from build123d import *

# Parameters (mm, degrees)
SKETCH1_R           = 2.375
BOSS_EXTRUDE1_DEPTH = 22.5
SKETCH2_R           = 1.6
BOSS_EXTRUDE2_DEPTH = 0.6
SKETCH3_R           = 2.375
BOSS_EXTRUDE3_DEPTH = 4.4


with BuildPart() as part:
    # Sketch1 → Boss-Extrude1 (new body)
    with BuildSketch(Plane.XY):
        with Locations(Location((0, 0, 0), (0, 0, 180))):
            Circle(SKETCH1_R)
    boss_extrude1 = extrude(amount=BOSS_EXTRUDE1_DEPTH)

    # Sketch2 → Boss-Extrude2 (add)
    with BuildSketch(Plane.XY.offset(22.5)):
        Circle(SKETCH2_R)
    boss_extrude2 = extrude(amount=BOSS_EXTRUDE2_DEPTH)

    # Sketch3 → Boss-Extrude3 (add)
    with BuildSketch(Plane.XY.offset(23.1)):
        with Locations(Location((0, 0, 0), (0, 0, 180))):
            Circle(SKETCH3_R)
    boss_extrude3 = extrude(amount=BOSS_EXTRUDE3_DEPTH)

    # Mirror1: Boss-Extrude1, Boss-Extrude2, Boss-Extrude3 across plane
    add(boss_extrude1.mirror(Plane.XY))
    add(boss_extrude2.mirror(Plane.XY))
    add(boss_extrude3.mirror(Plane.XY))


solid = part.part
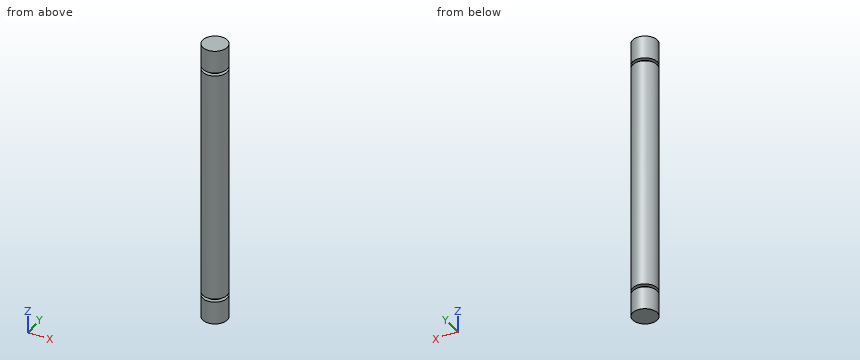
Build history of the part. All positions in model axes, mm. Give positions to 0.01 mm unless a question says otherwise; leave off trailing zeros. Order: outer loops, then holes, each group sorted by start corner. A loop starts at its lowest first (then second) coordinate and runs counter-clockwise, first axis right, second up. Notation, with made-up numbers: M -14.5,21 L 20.5,21 A20 cw 20.5,49 Z; hole C 71,69.5 d3. An arc over 180 degrees is marked long. Put each result on its own line as item: value.
Item 1: Slice it at C-C, the plane z = -17.5. Write the cut outline in (x, y) (3 decimals).
From the geometry:
outline: C 0,0 d4.75
Item 2: Slice it at B-B, the plane x = -1.05. Write the cut outline in (y, z).
From the geometry:
outline: M -2.13,-27.5 L 2.13,-27.5 L 2.13,-23.1 L 1.21,-23.1 L 1.21,-22.5 L 2.13,-22.5 L 2.13,22.5 L 1.21,22.5 L 1.21,23.1 L 2.13,23.1 L 2.13,27.5 L -2.13,27.5 L -2.13,23.1 L -1.21,23.1 L -1.21,22.5 L -2.13,22.5 L -2.13,-22.5 L -1.21,-22.5 L -1.21,-23.1 L -2.13,-23.1 Z
Item 3: Probe line 1 (Z direction, x = 1.9, y = 1.1); line 2 (X direction, y = 0.1, z = -1.5); line 3 (X direction, y = 0.4, z = -12.5). List the from-to ranges inside material, lowest first. Write a range as [from, to].
From the geometry:
line 1: z = [-27.5, -23.1], [-22.5, 22.5], [23.1, 27.5]
line 2: x = [-2.37, 2.37]
line 3: x = [-2.34, 2.34]
Item 4: Slice it at A-A, the plane y = 1. Write the cut outline in (x, z), plus the area to 3 significant figures.
From the geometry:
outline: M -2.15,-27.5 L 2.15,-27.5 L 2.15,-23.1 L 1.25,-23.1 L 1.25,-22.5 L 2.15,-22.5 L 2.15,22.5 L 1.25,22.5 L 1.25,23.1 L 2.15,23.1 L 2.15,27.5 L -2.15,27.5 L -2.15,23.1 L -1.25,23.1 L -1.25,22.5 L -2.15,22.5 L -2.15,-22.5 L -1.25,-22.5 L -1.25,-23.1 L -2.15,-23.1 Z
area: 235 mm2
